Can you work these out from the model? Positions are in its coordinate system, mm. Face numbers are marked on the shaded views. A direction names the side the tool comes from. Give positions to 0.01 mm unless a question says otherwise; leave off trailing zeros. Order: outer loops, then holes, each group sorted by start corner. A loop starts at its lowest first (then second) coordinate and runs counter-clockwise, first axis right, second up. Notation, with made-up numbers: (10.5, -1.75) - (31.5, -1.75) arc R20 ccw to (31.5, 2.25) - close; hole circle Ø3 at (89.5, -36.75). An arc over 180 degrees is marked (long way). Return JSON: item names as keys, results as strings.
```python
from build123d import *

# Parameters (mm, degrees)
SKETCH1_W           = 20.4
SKETCH1_H           = 41
BOSS_EXTRUDE1_DEPTH = 10
CUT_EXTRUDE1_REACH  = 69.823
SKETCH2_W           = 7
SKETCH2_H           = 10
SKETCH3_W           = 25
SKETCH3_H           = 5
BOSS_EXTRUDE2_DEPTH = 10


with BuildPart() as part:
    # Sketch1 → Boss-Extrude1 (new body)
    with BuildSketch(Plane.XY):
        with BuildLine():
            Line((-15, 24.5), (-15, -20.5))
            ThreePointArc((-15, -20.5), (-16.464466094, -24.035533906), (-20, -25.5))
            Line((-20, -25.5), (-30, -25.5))
            Line((-30, -25.5), (-30, -35.5))
            Line((-30, -35.5), (30, -35.5))
            Line((30, -35.5), (30, -25.5))
            Line((30, -25.5), (20, -25.5))
            ThreePointArc((20, -25.5), (16.464466094, -24.035533906), (15, -20.5))
            Line((15, -20.5), (15, 24.5))
            Line((15, 24.5), (-15, 24.5))
        make_face()
        Rectangle(SKETCH1_W, SKETCH1_H, mode=Mode.SUBTRACT)
    extrude(amount=BOSS_EXTRUDE1_DEPTH)

    # Sketch2 → Cut-Extrude1 (cut, up to next)
    with BuildSketch(Plane(origin=(0, 24.5, 0), x_dir=(1, 0, 0), z_dir=(0, 1, 0)), mode=Mode.PRIVATE) as cut_extrude1_sk1:
        with Locations((0, -5)):
            Rectangle(SKETCH2_W, SKETCH2_H)
    cut_extrude1_tool1 = extrude(cut_extrude1_sk1.sketch, amount=-CUT_EXTRUDE1_REACH, mode=Mode.PRIVATE) & part.part
    add(cut_extrude1_tool1.solids().sort_by_distance((0, 24.5, 5))[0], mode=Mode.SUBTRACT)

    # Sketch3 → Boss-Extrude2 (add)
    with BuildSketch(Plane.XY.offset(10)):
        with Locations((0, -33)):
            Rectangle(SKETCH3_W, SKETCH3_H)
    extrude(amount=BOSS_EXTRUDE2_DEPTH)


solid = part.part
```
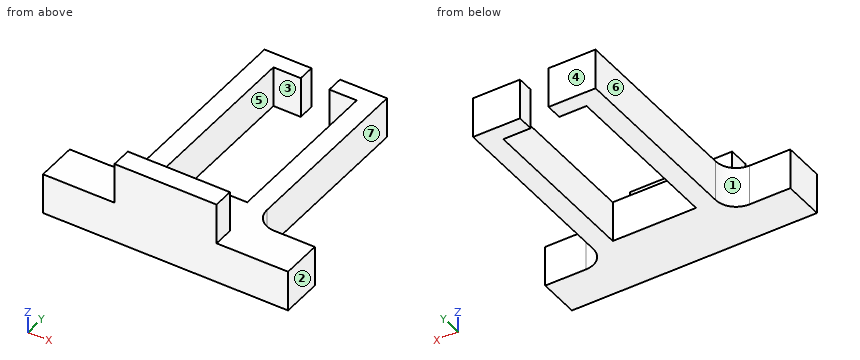
1. On a 3-axis mill with a long thin cutter (end or side, diameter ignored), from which of +Z, -Z, +X, -X, +Y, -Y can I reach the whole of each face in a straight line? I mean the marked faces 4, 5, 6 and 7. Say none if no direction works.
Checks:
{"face 4": "+Z, -Z, +X, -X, +Y", "face 5": "+Z, -Z", "face 6": "+Z, -Z, -X, +Y", "face 7": "+Z, -Z, +X, +Y"}
2. Suppose I cut it at B-B (z = 6). List the corners of the cut face in (x, y) for me, plus the area to 3 significant figures.
Checks:
{"outline": "(-30, -35.5) - (30, -35.5) - (30, -25.5) - (20, -25.5) arc R5 cw to (15, -20.5) - (15, 24.5) - (3.5, 24.5) - (3.5, 20.5) - (10.2, 20.5) - (10.2, -20.5) - (-10.2, -20.5) - (-10.2, 20.5) - (-3.5, 20.5) - (-3.5, 24.5) - (-15, 24.5) - (-15, -20.5) arc R5 cw to (-20, -25.5) - (-30, -25.5) - close", "area": "1,250 mm^2"}
3. If I drill on L1, parallel to X at y = 21, z = 4; L2, parallel to X at y = 9, z = 3.75; L3, parallel to Y at x = -9, z = 4, over which ranges is the centre line in solid material (lowest first)? Write a range as [from, to].
Checks:
{"L1": "[-15, -3.5], [3.5, 15]", "L2": "[-15, -10.2], [10.2, 15]", "L3": "[-35.5, -20.5], [20.5, 24.5]"}
4. Suppose I cut it at A-A (y = -4.5). List the corners of the cut face in (x, z) for me, plus the area to 3 significant figures.
Checks:
{"outline": "(-15, 0) - (-10.2, 0) - (-10.2, 10) - (-15, 10) - close; (10.2, 0) - (15, 0) - (15, 10) - (10.2, 10) - close", "area": "96.0 mm^2"}
5. Thinking about a two-plate mould opening in Y: for the marked faces 1, 2 and 3, which applies, +Y half, -Y half, draft (parallel to the pull), parting line (faces both ways), or undercut?
Checks:
{"face 1": "+Y half", "face 2": "draft", "face 3": "undercut"}
6. For pin 1 Ø1.5 at (y, z) = (-32, 14.5) entering from -X; pin 2 Ø3 at (x, y) = (-12, -12.5) entering from +Z; pin 3 Ø11 at (y, z) = (-1, 6) entering from -X, each with a flat end and sliding along its axis, tell me the tip position at first contact or that it passes through.
Checks:
{"pin 1": "x = -12.5", "pin 2": "z = 10", "pin 3": "x = -15"}
7. Suppose I cut it at C-C (x = -14). List the corners of the cut face in (y, z) for me, plus the area to 3 significant figures.
Checks:
{"outline": "(-35.5, 0) - (24.5, 0) - (24.5, 10) - (-35.5, 10) - close", "area": "600 mm^2"}
8. Suppose I cut it at D-D (z = 16). List the corners of the cut face in (x, y) for me, plus the area to 3 significant figures.
Checks:
{"outline": "(-12.5, -35.5) - (12.5, -35.5) - (12.5, -30.5) - (-12.5, -30.5) - close", "area": "125 mm^2"}
